Design review of the part built by this model. Coordinates are the model's own, in mm. A direction names the side the tool comes from. Give positions to 0.01 mm unless a question says otherwise; leave off trailing zeros. Write each loop counter-clockwise with the first axis right and the second up, starting at its lowest first coordinate (ties: lowest second). Pieces come first, ordered by that corner, then holes. Notation, with made-up numbers: (50, 25.5) -> (85, 25.5) arc R36 cw to (85, 62.5) -> close; hole circle Ø7 at (-7, -17). An arc over 180 degrees is marked (long way). Answer as a JSON object with one key per item and string values.
```python
from build123d import *

# Parameters (mm, degrees)
CROQUIS1_W              = 140
CROQUIS1_H              = 140
CROQUIS1_R              = 1.5
SALIENTE_EXTRUIR1_DEPTH = 0.5
CROQUIS2_R              = 1.75
CROQUIS2_W              = 100
CROQUIS2_H              = 100
CORTAR_EXTRUIR1_DEPTH   = 10
SALIENTE_EXTRUIR3_START = 2.7
CROQUIS3_W              = 144
CROQUIS3_H              = 144
CROQUIS3_R              = 1.75
CROQUIS3_W_2            = 100
CROQUIS3_H_2            = 100
SALIENTE_EXTRUIR3_DEPTH = 2.7
CROQUIS4_W              = 144
CROQUIS4_H              = 144
CROQUIS4_W_2            = 140
CROQUIS4_H_2            = 140
SALIENTE_EXTRUIR4_DEPTH = 0.5
CROQUIS5_W              = 144
CROQUIS5_H              = 144
CROQUIS5_R              = 1.75
CROQUIS5_W_2            = 100
CROQUIS5_H_2            = 100
SALIENTE_EXTRUIR5_DEPTH = 0.5


with BuildPart() as part:
    # Croquis1 → Saliente-Extruir1 (new body)
    with BuildSketch(Plane(origin=(0, 0, 0), x_dir=(1, 0, 0), z_dir=(0, 1, 0))):
        Rectangle(CROQUIS1_W, CROQUIS1_H)
        with Locations(Location((-61, 61, 0), (0, 0, 270))):
            Circle(CROQUIS1_R, mode=Mode.SUBTRACT)
        with Locations(Location((66, 61, 0), (0, 0, 270))):
            Circle(CROQUIS1_R, mode=Mode.SUBTRACT)
        with Locations(Location((66, -61, 0), (0, 0, 270))):
            Circle(CROQUIS1_R, mode=Mode.SUBTRACT)
        with Locations(Location((-61, -61, 0), (0, 0, 270))):
            Circle(CROQUIS1_R, mode=Mode.SUBTRACT)
        with Locations(Location((66, 30.5, 0), (0, 0, 270))):
            Circle(CROQUIS1_R, mode=Mode.SUBTRACT)
        with Locations(Location((66, -30.5, 0), (0, 0, 270))):
            Circle(CROQUIS1_R, mode=Mode.SUBTRACT)
        with Locations(Location((-30.5, -66, 0), (0, 0, 270))):
            Circle(CROQUIS1_R, mode=Mode.SUBTRACT)
        with Locations(Location((30.5, -66, 0), (0, 0, 270))):
            Circle(CROQUIS1_R, mode=Mode.SUBTRACT)
        with Locations(Location((-30.5, 66, 0), (0, 0, 90))):
            Circle(CROQUIS1_R, mode=Mode.SUBTRACT)
        with Locations(Location((30.5, 66, 0), (0, 0, 90))):
            Circle(CROQUIS1_R, mode=Mode.SUBTRACT)
        with Locations(Location((-66, 30.5, 0), (0, 0, 90))):
            Circle(CROQUIS1_R, mode=Mode.SUBTRACT)
        with Locations(Location((-66, -30.5, 0), (0, 0, 90))):
            Circle(CROQUIS1_R, mode=Mode.SUBTRACT)
    extrude(amount=SALIENTE_EXTRUIR1_DEPTH)

    # Croquis2 → Cortar-Extruir1 (cut)
    with BuildSketch(Plane(origin=(0, 0.5, 0), x_dir=(1, 0, 0), z_dir=(0, 1, 0))):
        with Locations(Location((66, 61, 0), (0, 0, 270))):
            Circle(CROQUIS2_R)
        with Locations(Location((-61, 61, 0), (0, 0, 270))):
            Circle(CROQUIS2_R)
        with Locations(Location((-61, -61, 0), (0, 0, 270))):
            Circle(CROQUIS2_R)
        with Locations(Location((66, -61, 0), (0, 0, 270))):
            Circle(CROQUIS2_R)
        Polygon((-28.906513257, 63.24), (-27.313026514, 66), (-28.906513257, 68.76), (-32.093486743, 68.76), (-33.686973486, 66), (-32.093486743, 63.24), align=None)
        Polygon((32.093486743, 63.24), (33.686973486, 66), (32.093486743, 68.76), (28.906513257, 68.76), (27.313026514, 66), (28.906513257, 63.24), align=None)
        Polygon((67.593486743, 27.74), (69.186973486, 30.5), (67.593486743, 33.26), (64.406513257, 33.26), (62.813026514, 30.5), (64.406513257, 27.74), align=None)
        Polygon((67.593486743, -33.26), (69.186973486, -30.5), (67.593486743, -27.74), (64.406513257, -27.74), (62.813026514, -30.5), (64.406513257, -33.26), align=None)
        Polygon((32.093486743, -68.76), (33.686973486, -66), (32.093486743, -63.24), (28.906513257, -63.24), (27.313026514, -66), (28.906513257, -68.76), align=None)
        Polygon((-28.906513257, -68.76), (-27.313026514, -66), (-28.906513257, -63.24), (-32.093486743, -63.24), (-33.686973486, -66), (-32.093486743, -68.76), align=None)
        Polygon((-64.406513257, -33.26), (-62.813026514, -30.5), (-64.406513257, -27.74), (-67.593486743, -27.74), (-69.186973486, -30.5), (-67.593486743, -33.26), align=None)
        Polygon((-64.406513257, 27.74), (-62.813026514, 30.5), (-64.406513257, 33.26), (-67.593486743, 33.26), (-69.186973486, 30.5), (-67.593486743, 27.74), align=None)
        Rectangle(CROQUIS2_W, CROQUIS2_H)
    extrude(amount=-CORTAR_EXTRUIR1_DEPTH, mode=Mode.SUBTRACT)

    # Croquis3 → Saliente-Extruir3 (add)
    with BuildSketch(Plane(origin=(0, 0.5, 0), x_dir=(1, 0, 0), z_dir=(0, 1, 0)).offset(SALIENTE_EXTRUIR3_START)):
        Rectangle(CROQUIS3_W, CROQUIS3_H)
        with Locations(Location((-61, -61, 0), (0, 0, 270))):
            Circle(CROQUIS3_R, mode=Mode.SUBTRACT)
        with Locations(Location((-61, 61, 0), (0, 0, 270))):
            Circle(CROQUIS3_R, mode=Mode.SUBTRACT)
        with Locations(Location((66, 61, 0), (0, 0, 270))):
            Circle(CROQUIS3_R, mode=Mode.SUBTRACT)
        with Locations(Location((66, -61, 0), (0, 0, 270))):
            Circle(CROQUIS3_R, mode=Mode.SUBTRACT)
        Rectangle(CROQUIS3_W_2, CROQUIS3_H_2, mode=Mode.SUBTRACT)
        Polygon((-33.686973486, -66), (-32.093486743, -68.76), (-28.906513257, -68.76), (-27.313026514, -66), (-28.906513257, -63.24), (-32.093486743, -63.24), align=None, mode=Mode.SUBTRACT)
        Polygon((-67.593486743, -33.26), (-64.406513257, -33.26), (-62.813026514, -30.5), (-64.406513257, -27.74), (-67.593486743, -27.74), (-69.186973486, -30.5), align=None, mode=Mode.SUBTRACT)
        Polygon((28.906513257, 63.24), (32.093486743, 63.24), (33.686973486, 66), (32.093486743, 68.76), (28.906513257, 68.76), (27.313026514, 66), align=None, mode=Mode.SUBTRACT)
        Polygon((-33.686973486, 66), (-32.093486743, 63.24), (-28.906513257, 63.24), (-27.313026514, 66), (-28.906513257, 68.76), (-32.093486743, 68.76), align=None, mode=Mode.SUBTRACT)
        Polygon((62.813026514, 30.5), (64.406513257, 27.74), (67.593486743, 27.74), (69.186973486, 30.5), (67.593486743, 33.26), (64.406513257, 33.26), align=None, mode=Mode.SUBTRACT)
        Polygon((67.593486743, -33.26), (69.186973486, -30.5), (67.593486743, -27.74), (64.406513257, -27.74), (62.813026514, -30.5), (64.406513257, -33.26), align=None, mode=Mode.SUBTRACT)
        Polygon((33.686973486, -66), (32.093486743, -63.24), (28.906513257, -63.24), (27.313026514, -66), (28.906513257, -68.76), (32.093486743, -68.76), align=None, mode=Mode.SUBTRACT)
        Polygon((-64.406513257, 27.74), (-62.813026514, 30.5), (-64.406513257, 33.26), (-67.593486743, 33.26), (-69.186973486, 30.5), (-67.593486743, 27.74), align=None, mode=Mode.SUBTRACT)
    extrude(amount=-SALIENTE_EXTRUIR3_DEPTH)

    # Croquis4 → Saliente-Extruir4 (add)
    with BuildSketch(Plane.XZ.offset(-0.5)):
        Rectangle(CROQUIS4_W, CROQUIS4_H)
        Rectangle(CROQUIS4_W_2, CROQUIS4_H_2, mode=Mode.SUBTRACT)
    extrude(amount=SALIENTE_EXTRUIR4_DEPTH)

    # Croquis5 → Saliente-Extruir5 (add)
    with BuildSketch(Plane.XZ):
        Rectangle(CROQUIS5_W, CROQUIS5_H)
        with Locations(Location((66, -61, 0), (0, 0, 90))):
            Circle(CROQUIS5_R, mode=Mode.SUBTRACT)
        with Locations(Location((-61, -61, 0), (0, 0, 90))):
            Circle(CROQUIS5_R, mode=Mode.SUBTRACT)
        with Locations(Location((66, 61, 0), (0, 0, 90))):
            Circle(CROQUIS5_R, mode=Mode.SUBTRACT)
        with Locations(Location((-61, 61, 0), (0, 0, 90))):
            Circle(CROQUIS5_R, mode=Mode.SUBTRACT)
        with Locations(Location((66, 30.5, 0), (0, 0, 270))):
            Circle(CROQUIS5_R, mode=Mode.SUBTRACT)
        with Locations(Location((30.5, 66, 0), (0, 0, 270))):
            Circle(CROQUIS5_R, mode=Mode.SUBTRACT)
        with Locations(Location((-30.5, 66, 0), (0, 0, 270))):
            Circle(CROQUIS5_R, mode=Mode.SUBTRACT)
        with Locations(Location((-66, 30.5, 0), (0, 0, 270))):
            Circle(CROQUIS5_R, mode=Mode.SUBTRACT)
        with Locations(Location((-66, -30.5, 0), (0, 0, 270))):
            Circle(CROQUIS5_R, mode=Mode.SUBTRACT)
        with Locations(Location((-30.5, -66, 0), (0, 0, 270))):
            Circle(CROQUIS5_R, mode=Mode.SUBTRACT)
        with Locations(Location((30.5, -66, 0), (0, 0, 270))):
            Circle(CROQUIS5_R, mode=Mode.SUBTRACT)
        with Locations(Location((66, -30.5, 0), (0, 0, 270))):
            Circle(CROQUIS5_R, mode=Mode.SUBTRACT)
        Rectangle(CROQUIS5_W_2, CROQUIS5_H_2, mode=Mode.SUBTRACT)
    extrude(amount=SALIENTE_EXTRUIR5_DEPTH)


solid = part.part
```
(1) For faces 1 (the flat face through (53, 3.2, 5)), 2 (the flat face through (-66, 2, 27.74)), 3 (the flat face through (50, 1, -1)), list the 3-axis set-ups (+Z, -Z, +X, -X, +Y, -Y) from which the entire face can be reached by the end or side of a thin tool; tool diameter is ignored.
Here are the results:
{"face 1": "+Z, -Z, +X, -X, +Y", "face 2": "+Y", "face 3": "+Y, -Y"}
(2) The part is to be moulded in two halves that separate along Z. For faces 4 (the cylindrical face through (31.026, -0.246, -67.669)), 5 (the flat face through (-1, -0.5, -63)), say which applies: +Z half, -Z half, draft (parallel to the pull), parting line (faces both ways), or undercut.
Here are the results:
{"face 4": "undercut", "face 5": "draft"}
(3) For line 1 along X through (y, z) = (-0.4, -66); line 2 along Z through (x, y) = (-61, 0.7); line 3 along Z through (x, y) = (-29.5, 0.45), list the stretches that pass through material, from the lowest coordinate up.
Here are the results:
{"line 1": "x = -72 to -32.25, -28.75 to 28.75, 32.25 to 72", "line 2": "z = -72 to -62.75, -59.25 to 59.25, 62.75 to 72", "line 3": "z = -72 to -68.76, -63.24 to -50, 50 to 63.24, 68.76 to 72"}
(4) We need section B-B, the plane y = 1.2. Give the number of separate pieces and of enclosed holes in the cut face, then the cut area to 3 significant figures.
Here are the results:
{"separate pieces": "1", "enclosed holes": "13", "area": "10,500 mm²"}
(5) Clearance check with flat-ended pins moving along their axes: pin 1 (1.7 mm diameter, centred on x = 31.5, z = 65.5, fed in from +Y); pin 2 (2 mm diameter, centred on x = -30.5, z = -66, fed in from +Y). State where each tip first meets the part, or that it passes through.
Here are the results:
{"pin 1": "stops at y = 0", "pin 2": "passes through"}
(6) We need section A-A, the plane z = -9.5. State the section outline as (x, y) points, then the cut area to 3 significant figures.
Here are the results:
{"outline": "(-72, -0.5) -> (-50, -0.5) -> (-50, 3.2) -> (-72, 3.2) -> close; (50, -0.5) -> (72, -0.5) -> (72, 3.2) -> (50, 3.2) -> close", "area": "163 mm²"}
